from build123d import *

# Parameters (mm, degrees)
ESQUISSE1_W             = 8
ESQUISSE1_H             = 8
ESQUISSE3_W             = 5.2
ESQUISSE3_H             = 5.2
ENL_V_MAT_EXTRU_1_DEPTH = 5.5


with BuildPart() as part:
    # Esquisse1 → Révolution2 (revolve)
    with BuildSketch(Plane(origin=(0, 0, 0), x_dir=(1, 0, 0), z_dir=(0, 1, 0)), mode=Mode.PRIVATE) as r_volution2_sk:
        with Locations((4, 4)):
            Rectangle(ESQUISSE1_W, ESQUISSE1_H)
    revolve(r_volution2_sk.sketch.rotate(Axis((0, 0, -8), (0, 0, 1)), 180), axis=Axis((0, 0, -8), (0, 0, 1)))

    # Esquisse3 → Enlèv. mat.-Extru.1 (cut)
    with BuildSketch(Plane.XY):
        Rectangle(ESQUISSE3_W, ESQUISSE3_H)
    extrude(amount=-ENL_V_MAT_EXTRU_1_DEPTH, mode=Mode.SUBTRACT)


solid = part.part
Work out the finished part from the listing and answer in its coordinate system (mm). A direction names the side the tool comes from. Coordinates: 2 decimals unless noted, no trailing zeros. Write each loop counter-clockwise with the first axis right and the second up, starting at its lowest first coordinate (ties: lowest second). Pieces come first, ordered by that corner, then holes.
1. The part is cut by section D-D, the plane z = -6.5. Write down the section's boundary in (x, y).
Results list:
outline: circle Ø16 at (0, 0)
2. The part is cut by section C-C, the plane z = -4.25. Write down the section's boundary in (x, y).
Results list:
outline: circle Ø16 at (0, 0); hole (-2.6, -2.6) - (2.6, -2.6) - (2.6, 2.6) - (-2.6, 2.6) - close
3. For a pull along Y with two mould halves and no side action, classify faces 1 (the cylindrical face through (1.73, 7.81, -4.06)), 2 (the flat face through (0, 0, -8)), 3 (the flat face through (2.6, 0, -3)) as +Y half, -Y half, draft (parallel to the pull), parting line (faces both ways), or undercut.
Results list:
face 1: parting line
face 2: draft
face 3: undercut
4. Flat-ended cylindrical pins translate along their axes: pin 1 (1 mm diameter, centred on x = -6, z = -3, fed in from +Y); pin 2 (1 mm diameter, centred on x = -1.5, z = -4.5, fed in from +Y); pin 3 (1.6 mm diameter, centred on x = 1.5, y = -1, fed in from +Z). Find the tip coordinate at first contact, or state that the pin passes through.
Results list:
pin 1: stops at y = 5.81
pin 2: stops at y = 7.94
pin 3: stops at z = -5.5
5. Consider line 1 along Y through (x, z) = (-0.25, -3.25); line 2 along X through (y, z) = (-2, -4.25). Determine where each line is inside the solid, lowest interval first.
Results list:
line 1: y = -8 to -2.6, 2.6 to 8
line 2: x = -7.75 to -2.6, 2.6 to 7.75
6. For faces 4 (the flat face through (0, 0, -5.5)), 5 (the flat face through (3, 0, 0)), determine the directions among +Z, -Z, +X, -X, +Y, -Y from which every point of the face is accessible in a straight line to the end or side of a thin tool.
Results list:
face 4: +Z
face 5: +Z, +X, -X, +Y, -Y
7. The part is cut by section A-A, the plane y = 0. Write down the section's boundary in (x, z).
Results list:
outline: (-8, -8) - (8, -8) - (8, 0) - (2.6, 0) - (2.6, -5.5) - (-2.6, -5.5) - (-2.6, 0) - (-8, 0) - close
